Can you work these out from the drawing? Everything is in mm from the part's minimum corner. Coordinates: 2 decimals unless noted, no trailing zeros. Write each loop counter-clockwise with the first axis right and the second up, starting at its lowest first coordinate (ties: lowest second). Pieces come first, ordered by that corner, then holes.
(1) Thinking about a two-plate mould opening in X: for the marked faces 1 and 2, which applies, released by +X, released by -X, zero draft, split by the parting line, or undercut?
(2) Please list where these lines run through material, in increasing order: probe 1 along X at (y, z) = (9.5, 36.5); probe 2 along Y at (x, z) = (11.25, 8); probe 3 along X at (y, z) = (13.75, 16.5).
(3) For pin 1 Ø4 at (y, z) = (7, 15.5) entering from -X; pin 2 Ø5 at (y, z) = (6.5, 35.5) entering from +X; pin 3 Ø1 at (x, y) = (11, 3) entering from -Z; pin 4 Ø7.5 at (x, y) = (9.525, 9.525) entering from -Z, each with a flat end and sliding along its axis, tell me the tip position at first contact or that it passes through.
(4) Imagine slicing it at A-A, the plane z = 27.5. List the corners of the cut face in (x, y) for me (3 decimals).
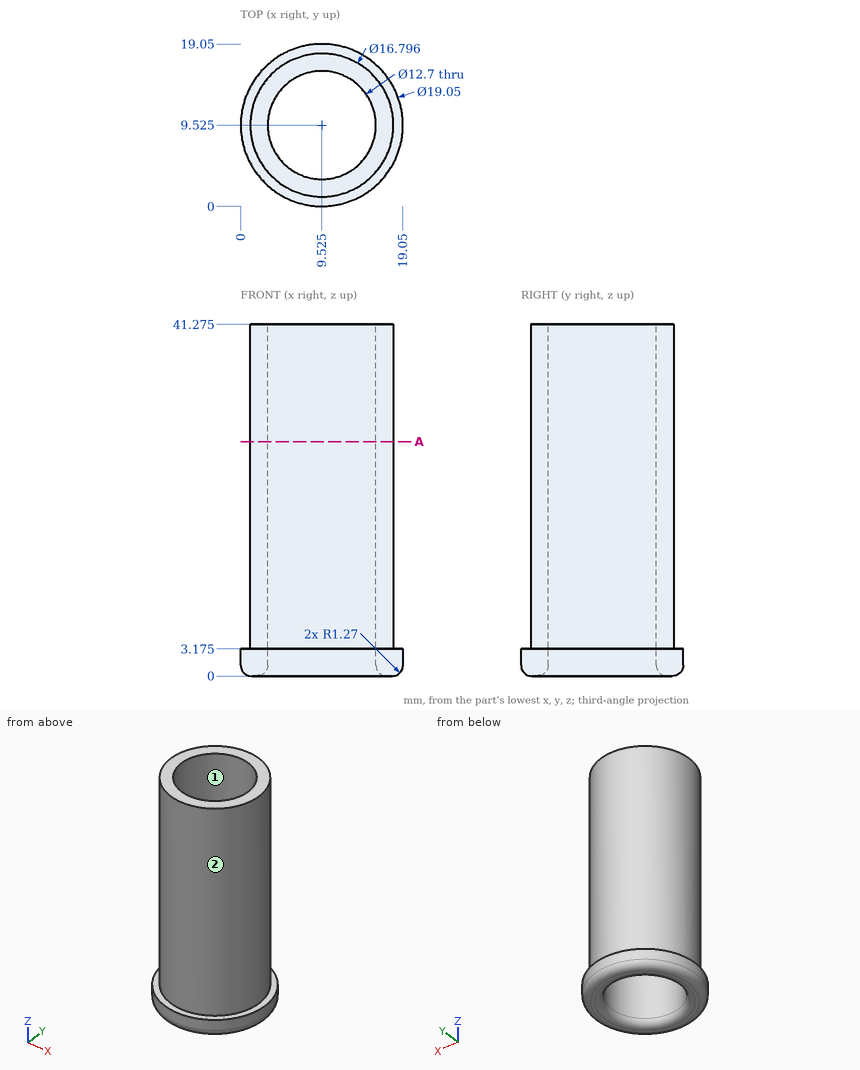
Recorded:
1. face 1: undercut
1. face 2: split by the parting line
2. probe 1: x = 1.13 to 3.18, 15.87 to 17.92
2. probe 2: y = 1.31 to 3.41, 15.64 to 17.74
2. probe 3: x = 2.27 to 4.78, 14.27 to 16.78
3. pin 1: stops at x = 1.14
3. pin 2: stops at x = 17.91
3. pin 3: stops at z = 0.08
3. pin 4: passes through
4. outline: circle Ø16.796 at (9.525, 9.525); hole circle Ø12.7 at (9.525, 9.525)
